The model under review builds one solid part; all positions refer to its coordinate system, in mm. Face numbers are marked on the shaded views. A direction names the side the tool comes from. Coordinates: 2 decimals unless noted, no trailing zeros. Loops run counter-clockwise (first coordinate to the right, second up) from the corner with the lowest first, then second, coordinate; pieces in that order, holes last. Notation, with made-up numbers: (89.25, 38.5) - (124.25, 38.5) arc R26 ccw to (124.25, 55.5) - close; hole circle Ø2 at (19.25, 51). An arc over 180 degrees is marked (long way). One line per item, written item: value. Start each with the question number.
1. Mouldability with a two-part tool opening along X and no side actions: class the marked faces 1 and 2 as +X half, -X half, draft (parallel to the pull), parting line (faces both ways), or undercut.
2. To check wall thickness, follow line 1 (X direction, y = 1.25, z = 1); line 2 (Y direction, x = 0, z = 4.5); line 3 (Y direction, x = -5.5, z = 6.5). State the ranges of each line that lie inside material, in increasing order.
3. We need section A-A, the plane y = 0. Give the boundary of the cut face in (x, z).
4. We need section D-D, the plane x = -10. Give the boundary of the cut face in (y, z).
5. For the marked faces 3, 4 and 5, list the 3-axis set-ups (+Z, -Z, +X, -X, +Y, -Y) from which the entire face can be reached by the end or side of a thin tool; tool diameter is ignored.
6. Insertion check: P1, Ø3, axis at y = -2, z = 3.5, coming from the -X side; P2, Ø4, axis at y = 3.5, z = 6, coming from the -X side; P3, Ø1.5, axis at x = -19.5, z = 1, coming from the -Y side. Each pin has a flat end and moves straight along its axis. Give the tip position at first contact, or say it passes through.
7. We need section C-C, the plane x = -50. Give the boundary of the cut face in (y, z), then the cut area to 3 significant figures.
8. We need section B-B, the plane z = 0.5. Give the boundary of the cut face in (x, y).
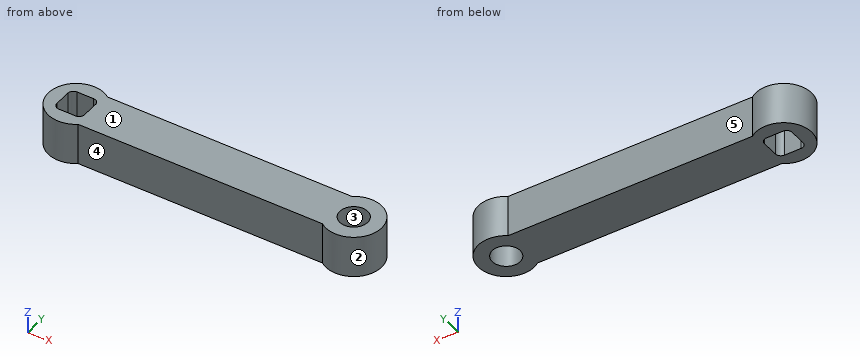
from build123d import *

# Parameters (mm, degrees)
SKETCH1_R           = 2.5
BOSS_EXTRUDE1_DEPTH = 7.5


with BuildPart() as part:
    # Sketch1 → Boss-Extrude1 (new body)
    with BuildSketch(Plane.XY):
        with BuildLine():
            Line((-47, 4), (-3, 4))
            ThreePointArc((-3, 4), (5, 0), (-3, -4))
            Line((-3, -4), (-47, -4))
            ThreePointArc((-47, -4), (-55, 0), (-47, 4))
        make_face()
        Circle(SKETCH1_R, mode=Mode.SUBTRACT)
        with BuildLine():
            Line((-51.5, -2.5), (-48.5, -2.5))
            ThreePointArc((-48.5, -2.5), (-47.792893219, -2.207106781), (-47.5, -1.5))
            Line((-47.5, -1.5), (-47.5, 1.5))
            ThreePointArc((-47.5, 1.5), (-47.792893219, 2.207106781), (-48.5, 2.5))
            Line((-48.5, 2.5), (-51.5, 2.5))
            ThreePointArc((-51.5, 2.5), (-52.207106781, 2.207106781), (-52.5, 1.5))
            Line((-52.5, 1.5), (-52.5, -1.5))
            ThreePointArc((-52.5, -1.5), (-52.207106781, -2.207106781), (-51.5, -2.5))
        make_face(mode=Mode.SUBTRACT)
    extrude(amount=BOSS_EXTRUDE1_DEPTH)


solid = part.part
Findings below:
1. face 1: draft
1. face 2: undercut
2. line 1: -54.84 to -52.5, -47.5 to -2.17, 2.17 to 4.84
2. line 2: -5 to -2.5, 2.5 to 5
2. line 3: -4 to 4
3. outline: (-55, 0) - (-52.5, 0) - (-52.5, 7.5) - (-55, 7.5) - close; (-47.5, 0) - (-2.5, 0) - (-2.5, 7.5) - (-47.5, 7.5) - close; (2.5, 0) - (5, 0) - (5, 7.5) - (2.5, 7.5) - close
4. outline: (-4, 0) - (4, 0) - (4, 7.5) - (-4, 7.5) - close
5. face 3: +Z, -Z
5. face 4: +Z, -Z, -Y
5. face 5: +Z, -Z, +Y
6. P1: x = -54.97
6. P2: x = -54.77
6. P3: y = -4
7. outline: (-5, 0) - (-2.5, 0) - (-2.5, 7.5) - (-5, 7.5) - close; (2.5, 0) - (5, 0) - (5, 7.5) - (2.5, 7.5) - close
7. area: 37.5 mm2
8. outline: (-47, -4) - (-3, -4) arc R5 ccw (long way) to (-3, 4) - (-47, 4) arc R5 ccw (long way) to start; hole (-52.5, -1.5) arc R1 ccw to (-51.5, -2.5) - (-48.5, -2.5) arc R1 ccw to (-47.5, -1.5) - (-47.5, 1.5) arc R1 ccw to (-48.5, 2.5) - (-51.5, 2.5) arc R1 ccw to (-52.5, 1.5) - close; hole circle Ø5 at (0, 0)
